Verification items for this drawing (mm, ordinates from the low corner). Give positions to 0.01 mm unless a question says otherwise; leave off trailing zeros. Loops run counter-clockwise (first coordinate to the right, second up) from the corner with the lowest first, then second, coordinate; pieces in that order, holes last. Notation, with made-up numbers: M 54,83 L 95,83 A23 cw 95,115 Z; hole C 76,43 d8. An arc over 180 degrees is marked long. Use one line per item in the form item = value.
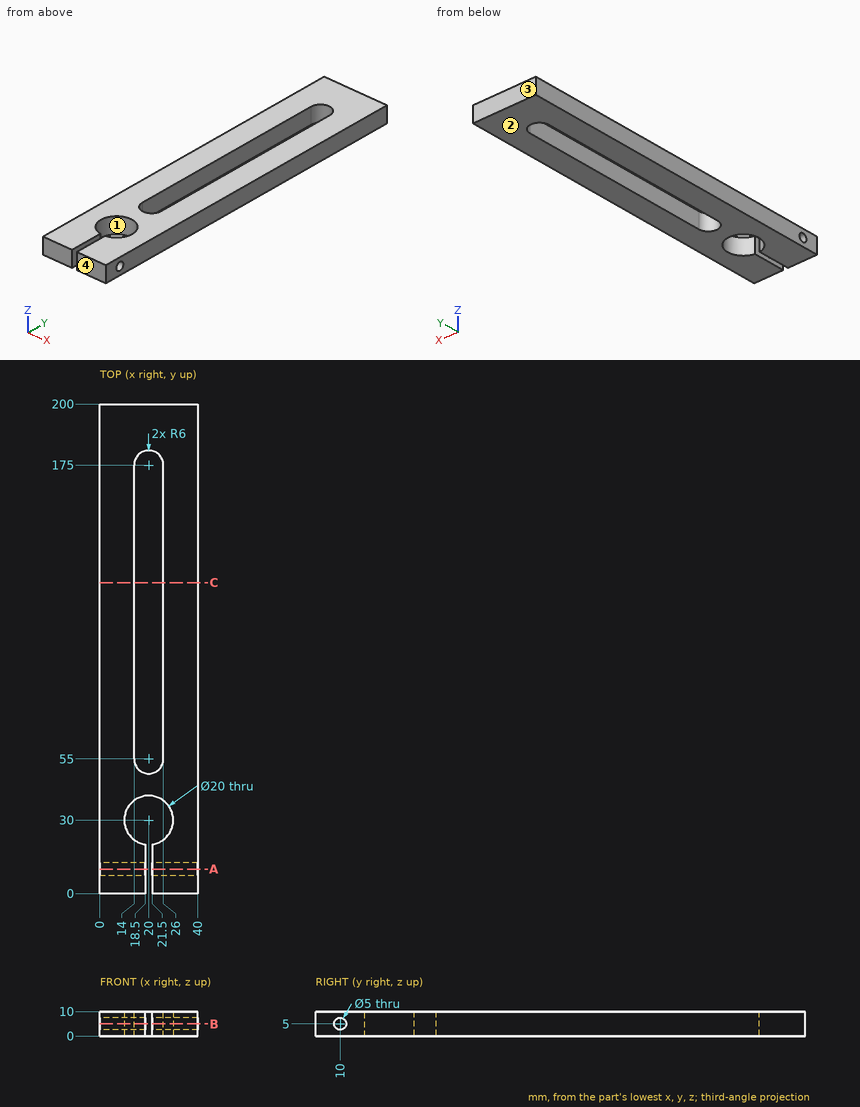
1) Release check for a two-part mould opening along Y. For the marked faces 1, 2, 3 and 4 record: pulls with the +Y half, pulls with the -Y half, needs draft (parallel to the pull), parting line crosses it, or undercut.
Evaluation:
face_1 = undercut
face_2 = needs draft
face_3 = pulls with the +Y half
face_4 = pulls with the -Y half
2) Scan lines: line 1 (X direction, y = 118.5, z = 8); line 2 (X direction, y = 30, z = 4.25); line 3 (Y direction, x = 27.5, z = 2.75). Record each from-to range of solid material in increasing order.
Evaluation:
line_1 = 0 to 14, 26 to 40
line_2 = 0 to 10, 30 to 40
line_3 = 0 to 8.91, 11.09 to 23.39, 36.61 to 200
3) Section check B-B (z = 5). Record the cut outline in (x, y), then the cut area to 3 significant figures.
Evaluation:
outline = M 0,0 L 18.5,0 L 18.5,7.5 L 0,7.5 Z; M 0,12.5 L 18.5,12.5 L 18.5,20.11 A10 cw long 21.5,20.11 L 21.5,12.5 L 40,12.5 L 40,200 L 0,200 Z; M 21.5,0 L 40,0 L 40,7.5 L 21.5,7.5 Z; hole M 14,55 A6 ccw 26,55 L 26,175 A6 ccw 14,175 Z
area = 5,890 mm^2
4) Depth check by flat-ended pin: pin 1 Ø1.5 at (x, y) = (5, 108) entering from -Z; pin 2 Ø4 at (y, z) = (10, 5) entering from +X. Enter the tip coordinate at first touch or a pass-through.
Evaluation:
pin_1 = 0
pin_2 = through
5) Section check C-C (y = 127). Record the cut outline in (x, z), then the cut area to 3 significant figures.
Evaluation:
outline = M 0,0 L 14,0 L 14,10 L 0,10 Z; M 26,0 L 40,0 L 40,10 L 26,10 Z
area = 280 mm^2
6) Section check A-A (y = 10). Record the cut outline in (x, z), then the cut area to 3 significant figures.
Evaluation:
outline = M 0,0 L 18.5,0 L 18.5,2.5 L 0,2.5 Z; M 0,7.5 L 18.5,7.5 L 18.5,10 L 0,10 Z; M 21.5,0 L 40,0 L 40,2.5 L 21.5,2.5 Z; M 21.5,7.5 L 40,7.5 L 40,10 L 21.5,10 Z
area = 185 mm^2
